```python
from build123d import *

# Parameters (mm, degrees)
F1_DEPTH    = 50
F2_T1_DEPTH = 66.3688124221


# Not quite as in the source:
# - a fillet or chamfer that OpenCascade refuses, or shapes differently, is made with other operations: its cross-section is extruded or revolved along the edge and cut away or added


with BuildPart() as f1:
    # F0 (on Front) → F1 (new body)
    with BuildSketch(Plane.XZ):
        with BuildLine():
            Line((7.5, 5), (0, 5))
            Line((0, 5), (-7.5, 5))
            Line((-7.5, 5), (-7.5, 0))
            Line((-7.5, 0), (-2.5, 0))
            ThreePointArc((-2.5, 0), (-1.767766953, 1.767766953), (0, 2.5))
            ThreePointArc((0, 2.5), (1.767766953, 1.767766953), (2.5, 0))
            Line((2.5, 0), (7.5, 0))
            Line((7.5, 0), (7.5, 5))
        make_face()
    extrude(amount=F1_DEPTH)

    # F2: chamfer of 5 on 2 edges, made by hand

    # F2_s2 → F2_t1 (cut)
    with BuildSketch(Plane.XZ.offset(-8.1844062111)):
        with BuildLine():
            Line((-5.5901699437, 0), (-1.8633899812, 1.6666666667))
            ThreePointArc((-1.8633899812, 1.6666666667), (-2.3064545677, 0.9645036688), (-2.5, 0))
            Line((-2.5, 0), (-5.5901699437, 0))
        make_face()
        with BuildLine():
            Line((5.5901699437, 0), (1.8633899812, 1.6666666667))
            ThreePointArc((1.8633899812, 1.6666666667), (2.3064545677, 0.9645036688), (2.5, 0))
            Line((2.5, 0), (5.5901699437, 0))
        make_face()
    extrude(amount=F2_T1_DEPTH, mode=Mode.SUBTRACT)


solid = f1.part
```
Work out the finished part from the listing and answer in its coordinate system (mm). A direction names the side the tool comes from. Round coordinates to 2 decimals unless told otherwise and drop trailing zeros. Write each loop counter-clockwise with the first axis right and the second up, starting at its lowest first coordinate (ties: lowest second). Pieces come first, ordered by that corner, then holes.
1) A cutting plane is placed at C-C on x = -0.5. Determine the outline of the cut face in (y, z), and give its area (3 significant figures).
2) A cutting plane is placed at A-A on z = 0.9. Determine the outline of the cut face in (x, y), and give its area (3 significant figures).
3) Consider probe 1 along X at (y, z) = (-2.5, 1.9); probe 2 along X at (y, z) = (-26, 1.55); probe 3 along Z at (x, y) = (-0.25, -13). Determine where each line is inside the solid, lowest interval first.
4) Which of the six approach directions +Z, -Z, +X, -X, +Y, -Y give full straight-line access (tool end or side, diameter ignored) to faces 4 (the face through (3.8, -24.7, 0.8)), 5 (the face through (-7, -25, 0))?
5) Determine the mould class of faces 1 (the face through (-7.5, -25, 3)), 2 (the face through (7, -25, 0)), 3 (the face through (-3.8, -24.7, 0.8)) for opening direction X: pulls with the +X half, pulls with the -X half, needs draft (parallel to the pull), parting line crosses it, or undercut.
6) A flat-ended cylindrical pin translates along its axis: P1, Ø5, axis at x = -5, y = -38.5, coming from the -Z side. Find the tip coordinate at first contact, or state that the pin passes through.
7) A cutting plane is placed at B-B on y = -12.5. Determine the outline of the cut face in (x, z).
Entries:
1. outline: (-50, 2.45) - (0, 2.45) - (0, 5) - (-50, 5) - close
1. area: 128 mm2
2. outline: (-7.5, -50) - (-3.58, -50) - (-3.58, 0) - (-7.5, 0) - close; (3.58, -50) - (7.5, -50) - (7.5, 0) - (3.58, 0) - close
2. area: 392 mm2
3. probe 1: x = -7.5 to -1.62, 1.62 to 7.5
3. probe 2: x = -7.5 to -2.12, 2.12 to 7.5
3. probe 3: z = 2.49 to 5
4. face 4: -Z, +Y, -Y
4. face 5: -Z, +X, -X, +Y, -Y
5. face 1: pulls with the -X half
5. face 2: needs draft
5. face 3: undercut
6. P1: stops at z = 0
7. outline: (-7.5, 0) - (-5.59, 0) - (-1.86, 1.67) arc R2.5 cw to (1.86, 1.67) - (5.59, 0) - (7.5, 0) - (7.5, 5) - (-7.5, 5) - close
